```python
from build123d import *

# Parameters (mm, degrees)
F3_D           = 5
F3_CSINK_D     = 13
F3_CSINK_ANGLE = 90


with BuildPart() as f1:
    # F0 (on Front) → F1 (revolve)
    with BuildSketch(Plane.XZ):
        with BuildLine():
            Line((-8, 0), (0, 0))
            Line((0, 0), (0, 13))
            Line((0, 13), (-10.5, 13))
            ThreePointArc((-10.5, 13), (-12.267767, 12.267767), (-13, 10.5))
            ThreePointArc((-13, 10.5), (-12.267767, 8.732233), (-10.5, 8))
            ThreePointArc((-10.5, 8), (-8.732233, 7.267767), (-8, 5.5))
            Line((-8, 5.5), (-8, 0))
        make_face()
    revolve(axis=Axis((0, 0, 6.5), (0, 0, -1)))

    # F3 (through all)
    with Locations(Plane.XY.offset(13)):
        with Locations((0, 0)):
            CounterSinkHole(F3_D / 2, F3_CSINK_D / 2, counter_sink_angle=F3_CSINK_ANGLE)


solid = f1.part
```
The model under review builds one solid part; all positions refer to its coordinate system, in mm. Coordinates: 2 decimals unless noted, no trailing zeros. Write each loop counter-clockwise with the first axis right and the second up, starting at its lowest first coordinate (ties: lowest second). Pieces come first, ordered by that corner, then holes. Notation, with made-up numbers: (-23, 76.25) - (16, 76.25) arc R33 cw to (16, 105.25) - close; hole circle Ø10 at (-21.5, 7). An arc over 180 degrees is marked (long way). Answer in a Markdown table with one row per item. Add a question column.
Q1. Draft analysis for pull direction Y (two halves, no side actions). For faces 1 (the face through (2, -2, 0)), 2 (the face through (1.73, -7.81, 2.71)), 3 (the face through (2.138, -1.639, 9.194)), state which applies: +Y half, -Y half, draft (parallel to the pull), parting line (faces both ways), or undercut.
Q2. To check wall thickness, follow line 1 along Y through (x, z) = (0, 4.25); line 2 along Y through (x, z) = (1.5, 0.5). State the ranges of each line that lie inside material, in increasing order. Write a range as from..to.
Q3. Consider section A-A on x = 0. Give the boundary of the cut face in (y, z), then the cut area to 3 significant figures.
Q4. Consider section D-D on z = 10. Give the boundary of the cut face in (x, y), then the cut area to 3 significant figures.
Q5. Consider section C-C on z = 3.5. Give the boundary of the cut face in (x, y), then the cut area to 3 significant figures.
Q6. Clearance check with flat-ended pins moving along their axes: pin 1 (3 mm diameter, centred on y = -10.5, z = 4.5, fed in from -X); pin 2 (2 mm diameter, centred on y = 4.5, z = 10, fed in from -X); pin 3 (1.5 mm diameter, centred on x = -7.5, y = -9.5, fed in from -Z); pin 4 (2 mm diameter, centred on x = -8.5, z = 7.5, fed in from +Y). State where each tip first meets the part, or that it passes through.
Answers below:
| question | item | result |
|---|---|---|
| 1 | face 1 | draft |
| 1 | face 2 | parting line |
| 1 | face 3 | undercut |
| 2 | line 1 | -8..-2.5, 2.5..8 |
| 2 | line 2 | -7.86..-2, 2..7.86 |
| 3 | outline | (-10.5, 8) arc R2.5 cw to (-8, 5.5) - (-8, 0) - (-2.5, 0) - (-2.5, 9) - (-6.5, 13) - (-10.5, 13) arc R2.5 ccw to start; (2.5, 0) - (8, 0) - (8, 5.5) arc R2.5 cw to (10.5, 8) arc R2.5 ccw to (10.5, 13) - (6.5, 13) - (2.5, 9) - close |
| 3 | area | 174 mm² |
| 4 | outline | circle Ø25.9 at (0, 0); hole circle Ø7 at (0, 0) |
| 4 | area | 488 mm² |
| 5 | outline | circle Ø16 at (0, 0); hole circle Ø5 at (0, 0) |
| 5 | area | 181 mm² |
| 6 | pin 1 | through |
| 6 | pin 2 | x = -12.5 |
| 6 | pin 3 | z = 8.15 |
| 6 | pin 4 | y = 8.69 |
